from build123d import *

# Parameters (mm, degrees)
SKETCH1_R           = 50
BOSS_EXTRUDE1_DEPTH = 40
FILLET1_R           = 5
SKETCH2_R           = 20
BOSS_EXTRUDE2_DEPTH = 20
SKETCH7_R           = 16.5
CUT_EXTRUDE1_DEPTH  = 20


with BuildPart() as part:
    # Sketch1 → Boss-Extrude1 (new, symmetric)
    with BuildSketch(Plane(origin=(0, 0, 0), x_dir=(1, 0, 0), z_dir=(0, 1, 0))):
        with BuildLine():
            Line((-60, 0), (-60, 80))
            Line((-60, 80), (60, 80))
            Line((60, 80), (60, 0))
            ThreePointArc((60, 0), (0, -60), (-60, 0))
        make_face()
        with Locations(Location((0, 0, 0), (0, 0, 270))):
            Circle(SKETCH1_R, mode=Mode.SUBTRACT)
    extrude(amount=BOSS_EXTRUDE1_DEPTH, both=True)

    # Fillet1
    fillet1_edges = [part.edges().sort_by_distance(p)[0] for p in [
        (-60, 0, -80),
        (60, 0, -80),
    ]]
    fillet(fillet1_edges, radius=FILLET1_R)

    # Sketch2 → Boss-Extrude2 (add)
    with BuildSketch(Plane(origin=(0, 0, -80), x_dir=(-1, 0, 0), z_dir=(0, 0, -1))):
        with Locations(Location((0, 0, 0), (0, 0, 180))):
            Circle(SKETCH2_R)
    extrude(amount=BOSS_EXTRUDE2_DEPTH)

    # Sketch7 → Cut-Extrude1 (cut)
    with BuildSketch(Plane(origin=(0, 0, -100), x_dir=(-1, 0, 0), z_dir=(0, 0, -1))):
        Circle(SKETCH7_R)
    extrude(amount=-CUT_EXTRUDE1_DEPTH, mode=Mode.SUBTRACT)


solid = part.part
Model file for the job. Use its own axes, mm. A direction names the side the tool comes from. Give positions to 0.01 mm unless a question says otherwise; leave off trailing zeros. Write each loop counter-clockwise with the first axis right and the second up, starting at its lowest first coordinate (ties: lowest second). Pieces come first, ordered by that corner, then holes. Notation, with made-up numbers: M -25.75,30.5 L 32.25,30.5 A20 ccw 32.25,66.5 Z; hole C -4,13 d10. An arc over 180 degrees is marked long. One line per item, written item: value. Start each with the question number.
Q1. Drop flat-ended pins along their axis: pin 1 Ø6 at (x, y) = (-25, -11.5) entering from -Z; pin 2 Ø3 at (x, y) = (-38.5, 16) entering from +Z; pin 3 Ø1.5 at (y, z) = (16.5, 5.5) entering from +X. Give the stop position or say it passes through.
Q2. Saw through at A-A, the plane x = 0. Write the cut outline in (y, z).
Q3. Saw through at D-D, the plane x = 42.5. Write the cut outline in (y, z), plus the area to 3 significant figures.
Q4. Saw through at B-B, the plane y = 0. Write the cut outline in (x, z), plus the area to 3 significant figures.
Q5. Probe probe 1 along Z at (x, y) = (-0.5, -4); probe 2 along Z at (x, y) = (44, 3.5); probe 3 along X at (y, z) = (-32.5, -6.5). List the from-to ranges inside material, lowest first. Write a range as [from, to].
Q6. Saw through at C-C, the plane z = 41.5. Write the cut outline in (x, y), plus the area to 3 significant figures.
Q7. 3-axis set-ups, long thin cutter, end or side, ignore diameter. For faces 1 (the flat face through (0, 0, -80)), 2 (the flat face through (1, 40, -58)): which of +Z, -Z, +X, -X, +Y, -Y reach the whole face in a straight line?
Q8. Two-plate mould, pull along Z, no slides. Class faces 3 (the flat face through (60, 1, -38)), 4 (the cylindrical face through (1.319, 0.56, 59.985)), 5 (the cylindrical face through (15.02, -0.56, 47.69)): +Z half, -Z half, draft (parallel to the pull), parting line (faces both ways), or undercut.
Output values:
1. pin 1: stops at z = -80
1. pin 2: stops at z = 47.23
1. pin 3: stops at x = 59.81
2. outline: M -40,-80 L -20,-80 L -20,-100 L -16.5,-100 L -16.5,-80 L 16.5,-80 L 16.5,-100 L 20,-100 L 20,-80 L 40,-80 L 40,-50 L -40,-50 Z; M -40,50 L 40,50 L 40,60 L -40,60 Z
3. outline: M -40,-80 L 40,-80 L 40,-26.34 L -40,-26.34 Z; M -40,26.34 L 40,26.34 L 40,42.35 L -40,42.35 Z
3. area: 5,570 mm²
4. outline: M -60,-75 A5 ccw -55,-80 L -20,-80 L -20,-100 L -16.5,-100 L -16.5,-80 L 16.5,-80 L 16.5,-100 L 20,-100 L 20,-80 L 55,-80 A5 ccw 60,-75 L 60,0 A60 ccw -60,0 Z; hole C 0,0 d100
4. area: 7,530 mm²
5. probe 1: z = [-80, -50], [50, 60]
5. probe 2: z = [-80, -23.75], [23.75, 40.79]
5. probe 3: x = [-60, -49.58], [49.58, 60]
6. outline: M -43.33,-40 L -27.89,-40 L -27.89,40 L -43.33,40 Z; M 27.89,-40 L 43.33,-40 L 43.33,40 L 27.89,40 Z
6. area: 2,470 mm²
7. face 1: -Z
7. face 2: +Z, -Z, +X, -X, +Y
8. face 3: draft
8. face 4: +Z half
8. face 5: undercut
